Can you work these out from the model? Positions are in its coordinate system, mm. Face numbers are marked on the shaded views. A direction names the side the tool comes from. Give positions to 0.01 mm unless a question says otherwise; leave off trailing zeros. Order: outer loops, then holes, each group sorted by start corner. A loop starts at its lowest first (then second) coordinate and runs counter-clockwise, first axis right, second up. Notation, with made-up numbers: (-1.75, 16.5) - (28.25, 16.5) arc R27 ccw to (28.25, 35.5) - close; hole circle Ø2 at (-12, 63). An arc over 180 degrees is marked (long way). Answer as CSV lines item,"result".
```python
from build123d import *

# Parameters (mm, degrees)
F4_D     = 5
F5_D     = 4.2
F5_DEPTH = 9.9705
F6_D     = 4.2


with BuildPart() as f1:
    # F0 (on Front) → F1 (revolve)
    with BuildSketch(Plane.XZ):
        Polygon((5.5753, 20.0152), (5.5753, 0), (9.652, 0), (9.652, 26.416), (9.9695, 26.416), (9.9695, 33.5534), (7.4295, 36.0934), (5.0165, 36.0934), (5.0165, 25.0444), (0, 25.0444), (0, 20.0152), align=None)
    revolve(axis=Axis((0, 0, 18.0467), (0, 0, 1)))

    # F4 (through all)
    with Locations(Plane.XY.offset(25.0444)):
        with Locations((0, 0)):
            Hole(F4_D / 2)

    # F5 (through all, one way)
    with BuildSketch(Plane.YZ):
        with Locations((0, 14.2)):
            Circle(F5_D / 2)
    extrude(amount=-F5_DEPTH, mode=Mode.SUBTRACT)

    # F6 (through all)
    with Locations(Plane(origin=(0, 0, 0), x_dir=(0, 1, 0), z_dir=(-1, 0, 0))):
        with Locations((0, -14.2)):
            Hole(F6_D / 2)


solid = f1.part
```
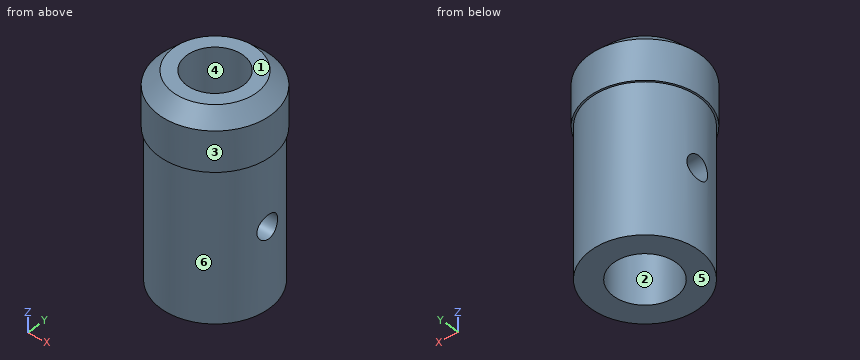
1) Which directions (+Z, -Z, +X, -X, +Y, -Y) give clear straight access to the entire face, cutting with the end or side of a thin tool? Please do the marked faces 4, 5 and 6.
Answer block:
face 4,"+Z"
face 5,"-Z, +X, -X, +Y, -Y"
face 6,"-Z"
2) I want a section at C-C on z = 19. Write out the boundary of the cut face in (x, y), plus the area to 3 significant figures.
Answer block:
outline,"circle Ø19.3 at (0, 0); hole circle Ø11.15 at (0, 0)"
area,"195 mm2"
3) I want a section at B-B on z = 14.2. Write out the boundary of the cut face in (x, y), plus the area to 3 significant figures.
Answer block:
outline,"(-9.42, -2.1) arc R9.65 ccw to (9.42, -2.1) - (5.16, -2.1) arc R5.58 cw to (-5.16, -2.1) - close; (-9.42, 2.1) - (-5.16, 2.1) arc R5.58 cw to (5.16, 2.1) - (9.42, 2.1) arc R9.65 ccw to start"
area,"160 mm2"
4) I need wall thicknesses on line 1 along Y through (x, z) = (0, 3); line 2 along Y through (x, z) = (6.75, 14.2); line 3 along X through (y, z) = (0.75, 25). Which ranges of each line are inside material? Lowest first, please. Write a range as [from, to].
Answer block:
line 1,"[-9.65, -5.58], [5.58, 9.65]"
line 2,"[-6.9, -2.1], [2.1, 6.9]"
line 3,"[-9.62, -2.38], [2.38, 9.62]"
5) I want a section at D-D on z = 25.5. Write out the boundary of the cut face in (x, y), plus the area to 3 significant figures.
Answer block:
outline,"circle Ø19.3 at (0, 0); hole circle Ø10.03 at (0, 0)"
area,"214 mm2"
6) If we mould it in two halves opening along Y, with no side actions, what happens to the marked faces 1, 2 and 3? For each: +Y half, -Y half, draft (parallel to the pull), parting line (faces both ways), or undercut.
Answer block:
face 1,"draft"
face 2,"undercut"
face 3,"parting line"
7) I'm going to push flat-ended pins straight in: P1, Ø5, axis at x = 0, y = -1, coming from the +Z side; P2, Ø3, axis at x = 0, y = 0, coming from the +Z side; P3, Ø6, axis at y = -5.5, z = 19.5, coming from the +X side; P4, Ø6, axis at x = -2.5, z = 21, coming from the -Y side. Where does each tip first touch, or does it pass through?
Answer block:
P1,"z = 25.04"
P2,"through"
P3,"x = 9.32"
P4,"y = -9.65"
8) I want a section at A-A on x = 0. Write out the boundary of the cut face in (y, z), plus the area to 3 significant figures.
Answer block:
outline,"(-9.97, 26.42) - (-9.65, 26.42) - (-9.65, 0) - (-5.58, 0) - (-5.58, 20.02) - (-2.5, 20.02) - (-2.5, 25.04) - (-5.02, 25.04) - (-5.02, 36.09) - (-7.43, 36.09) - (-9.97, 33.55) - close; (2.5, 20.02) - (5.58, 20.02) - (5.58, 0) - (9.65, 0) - (9.65, 26.42) - (9.97, 26.42) - (9.97, 33.55) - (7.43, 36.09) - (5.02, 36.09) - (5.02, 25.04) - (2.5, 25.04) - close"
area,"337 mm2"
